```python
from build123d import *

# Parameters (mm, degrees)
PAD_DEPTH    = 62
FILLET_R     = 1
SKETCH001_W  = 10
SKETCH001_H  = 11
PAD001_DEPTH = 5


with BuildPart() as part:
    # Sketch (on XY_Plane of Origin) → Pad (new body)
    with BuildSketch(Plane.XY):
        Polygon((23.094011, 0), (-11.547005, 20), (-11.547005, -20), align=None)
    extrude(amount=PAD_DEPTH)

    # Fillet
    fillet_edges = [part.edges().sort_by_distance(p)[0] for p in [
        (-11.547005, 20, 31),
        (23.094011, 0, 31),
        (-11.547005, -20, 31),
    ]]
    fillet(fillet_edges, radius=FILLET_R)

    # Sketch001 (on Face5 of Fillet) → Pad001 (join)
    with BuildSketch(Plane.XY.offset(62)):
        with Locations((-6.547005, 0)):
            Rectangle(SKETCH001_W, SKETCH001_H)
    extrude(amount=PAD001_DEPTH)


solid = part.part
```
Input: part model. Units: mm. Frame: model coordinates. A direction names the side the tool comes from. Round coordinates to 2 decimals unless told otherwise and drop trailing zeros. Order: outer loops, then holes, each group sorted by start corner. A loop starts at its lowest first (then second) coordinate and runs counter-clockwise, first axis right, second up. Notation, with made-up numbers: (62.25, -33) - (119.25, -33) arc R19 ccw to (119.25, -3) - close; hole circle Ø11 at (43, 32.25). An arc over 180 degrees is marked (long way). One line per question, with ' | ' between items. Start each with the question number.
1) Cut plane A-A, the plane x = -2.5. Return the cut outline in (y, z).
2) Cut plane C-C, the plane y = -13. Return the cut outline in (x, z), then the cut area to 3 significant figures.
3) Cut plane D-D, the plane x = -8. Return the cut outline in (y, z).
4) Ray query, probe 1 along Z at (x, y) = (-2, -14); probe 2 along Y at (x, z) = (15.5, 42.5); probe 3 along Y at (x, z) = (8, 49.5). Return the intervals inside material, ascending.
5) Contact query for flat-ended pins moving along their axis: P1, Ø5, axis at x = -2.5, y = -11.5, coming from the -Z side; P2, Ø12, axis at x = 17.5, z = 57.5, coming from the -Y side; P3, Ø5.5, axis at x = -5.5, z = 64.5, coming from the -Y side; P4, Ø1.5, axis at x = -6.5, z = 64.5, coming from the +Y side. Output: stop coordinate, or through.
6) Cut plane B-B, the plane z = 44. Return the cut outline in (x, y), then the cut area to 3 significant figures.
7) Set-up query: faces 1 (the flat face through (-1.547, 0, 64)), 2 (the flat face through (-7, 5.5, 64)), 3 (the flat face through (-7, -5.5, 64)). Return all of +Z, -Z, +X, -X, +Y, -Y with unobstructed straight access to the full face (end or side cutting, diameter ignored); none if empty.
Worked out:
1) outline: (-14.78, 0) - (14.78, 0) - (14.78, 62) - (5.5, 62) - (5.5, 67) - (-5.5, 67) - (-5.5, 62) - (-14.78, 62) - close
2) outline: (-11.55, 0) - (0.58, 0) - (0.58, 62) - (-11.55, 62) - close | area: 752 mm^2
3) outline: (-17.95, 0) - (17.95, 0) - (17.95, 62) - (5.5, 62) - (5.5, 67) - (-5.5, 67) - (-5.5, 62) - (-17.95, 62) - close
4) probe 1: z = 0 to 62 | probe 2: y = -4.38 to 4.38 | probe 3: y = -8.71 to 8.71
5) P1: stops at z = 0 | P2: stops at y = -6.69 | P3: stops at y = -17.17 | P4: stops at y = 5.5
6) outline: (-11.55, -18.27) arc R1 ccw to (-10.05, -19.13) - (21.59, -0.87) arc R1 ccw to (21.59, 0.87) - (-10.05, 19.13) arc R1 ccw to (-11.55, 18.27) - close | area: 691 mm^2
7) face 1: +Z, +X, +Y, -Y | face 2: +Z, +X, -X, +Y | face 3: +Z, +X, -X, -Y
